from build123d import *

# Parameters (mm, degrees)
BOSS_EXTRUDE1_DEPTH = 6.35
SKETCH2_R           = 1.27
CUT_EXTRUDE1_DEPTH  = 397.811495062
SKETCH5_R           = 1.27
CUT_EXTRUDE2_DEPTH  = 397.811495062
SKETCH6_W           = 38.1
SKETCH6_H           = 7.62
CUT_EXTRUDE5_DEPTH  = 397.811495062
CUT_EXTRUDE9_DEPTH  = 397.811495062
SKETCH15_W          = 22.606
SKETCH15_H          = 12.446
CUT_EXTRUDE12_DEPTH = 397.811495062
SKETCH17_R          = 1.1
CUT_EXTRUDE13_DEPTH = 343.418665957
SKETCH18_R          = 1.5875
SKETCH18_R_2        = 1.5
SKETCH18_R_3        = 1.651
CUT_EXTRUDE14_DEPTH = 343.36317383
SKETCH19_R          = 1.65
CUT_EXTRUDE15_DEPTH = 343.36317383
SKETCH20_R          = 11.43
CUT_EXTRUDE16_DEPTH = 397.811495062
SKETCH24_R          = 1.905
CUT_EXTRUDE20_DEPTH = 343.36317383


with BuildPart() as part:
    # Sketch1 → Boss-Extrude1 (new body)
    with BuildSketch(Plane(origin=(0, 0, 0), x_dir=(1, 0, 0), z_dir=(0, 1, 0))):
        with BuildLine():
            Line((-203.2, 0), (-50.8, 0))
            ThreePointArc((-50.8, 0), (-14.878975516, 14.878975516), (0, 50.8))
            Line((0, 50.8), (0, 132.097510542))
            add(Edge.make_bspline(
                [(0, 132.097510542), (-11.235039637, 303.015237559), (-127, 304.8)],
                knots=[0.173908828, 0.173908828, 0.173908828, 0.982925822, 0.982925822, 0.982925822], degree=2))
            add(Edge.make_bspline(
                [(-254, 132.097510542), (-242.764960363, 303.015237559), (-127, 304.8)],
                knots=[0.173908828, 0.173908828, 0.173908828, 0.982925822, 0.982925822, 0.982925822], degree=2))
            Line((-254, 132.097510542), (-254, 50.8))
            ThreePointArc((-254, 50.8), (-239.121024484, 14.878975516), (-203.2, 0))
        make_face()
    extrude(amount=BOSS_EXTRUDE1_DEPTH)

    # Sketch2 → Cut-Extrude1 (cut, through all)
    with BuildSketch(Plane(origin=(0, 6.35, 0), x_dir=(1, 0, 0), z_dir=(0, 1, 0))):
        with Locations(Location((-135.34380131, 269.24, 0), (0, 0, 270))):
            Circle(SKETCH2_R)
    extrude(amount=-CUT_EXTRUDE1_DEPTH, mode=Mode.SUBTRACT)

    # Sketch5 → Cut-Extrude2 (cut, through all)
    with BuildSketch(Plane(origin=(0, 6.35, 0), x_dir=(1, 0, 0), z_dir=(0, 1, 0))):
        with Locations(Location((-119.59580131, 269.24, 0), (0, 0, 270))):
            Circle(SKETCH5_R)
    extrude(amount=-CUT_EXTRUDE2_DEPTH, mode=Mode.SUBTRACT)

    # Sketch6 → Cut-Extrude5 (cut, through all)
    with BuildSketch(Plane(origin=(0, 6.35, 0), x_dir=(1, 0, 0), z_dir=(0, 1, 0))):
        with Locations((-158.75, 207.01)):
            Rectangle(SKETCH6_W, SKETCH6_H)
        with Locations((-158.75, 260.35)):
            Rectangle(SKETCH6_W, SKETCH6_H)
        with Locations((-95.25000011, 207.01)):
            Rectangle(SKETCH6_W, SKETCH6_H)
        with Locations((-95.25000011, 260.35)):
            Rectangle(SKETCH6_W, SKETCH6_H)
    extrude(amount=-CUT_EXTRUDE5_DEPTH, mode=Mode.SUBTRACT)

    # Sketch12 → Cut-Extrude9 (cut, through all)
    with BuildSketch(Plane(origin=(0, 6.35, 0), x_dir=(1, 0, 0), z_dir=(0, 1, 0))):
        with BuildLine():
            Line((-152.4, 125.095), (-101.6, 125.095))
            ThreePointArc((-101.6, 125.095), (-99.695, 127), (-101.6, 128.905))
            Line((-101.6, 128.905), (-152.4, 128.905))
            ThreePointArc((-152.4, 128.905), (-154.305, 127), (-152.4, 125.095))
        make_face()
        Polygon((-159.512, 101.6), (-159.512, 88.9), (-145.203610871, 88.9), (-94.5, 88.9), (-94.5, 101.6), align=None)
    extrude(amount=-CUT_EXTRUDE9_DEPTH, mode=Mode.SUBTRACT)

    # Sketch15 → Cut-Extrude12 (cut, through all)
    with BuildSketch(Plane(origin=(0, 6.35, 0), x_dir=(1, 0, 0), z_dir=(0, 1, 0))):
        with Locations((-127.000000055, 25.4)):
            Rectangle(SKETCH15_W, SKETCH15_H)
    extrude(amount=-CUT_EXTRUDE12_DEPTH, mode=Mode.SUBTRACT)

    # Sketch17 → Cut-Extrude13 (cut, through all)
    with BuildSketch(Plane(origin=(-70.897607534, -2.5, -15.584277619), x_dir=(1, 0, 0), z_dir=(0, -1, 0))):
        with Locations(Location((-70.055392521, -9.692722381, 0), (0, 0, 270))):
            Circle(SKETCH17_R)
        with Locations(Location((-42.255392521, -9.692722381, 0), (0, 0, 90))):
            Circle(SKETCH17_R)
    extrude(amount=-CUT_EXTRUDE13_DEPTH, mode=Mode.SUBTRACT)

    # Sketch18 → Cut-Extrude14 (cut, through all)
    with BuildSketch(Plane(origin=(-70.897607534, 6.35, -15.584277619), x_dir=(1, 0, 0), z_dir=(0, -1, 0))):
        with Locations(Location((-108.366177987, -107.537321923, 0), (0, 0, 270))):
            Circle(SKETCH18_R)
        with Locations(Location((-156.626177987, -108.807321923, 0), (0, 0, 270))):
            Circle(SKETCH18_R)
        with Locations(Location((-141.386177987, -159.607321923, 0), (0, 0, 270))):
            Circle(SKETCH18_R)
        with Locations(Location((-113.446177987, -159.607321923, 0), (0, 0, 270))):
            Circle(SKETCH18_R)
        with Locations(Location((-36.13742283, -36.50630685, 0), (0, 0, 270))):
            Circle(SKETCH18_R_2)
        with Locations(Location((-76.13742283, -55.50630685, 0), (0, 0, 270))):
            Circle(SKETCH18_R_2)
        with Locations(Location((-82.468497304, -27.730722381, 0), (0, 0, 270))):
            Circle(SKETCH18_R_3)
        with Locations(Location((-29.128497304, -27.730722381, 0), (0, 0, 270))):
            Circle(SKETCH18_R_3)
    extrude(amount=CUT_EXTRUDE14_DEPTH, mode=Mode.SUBTRACT)

    # Sketch19 → Cut-Extrude15 (cut, through all)
    with BuildSketch(Plane(origin=(-70.897607534, 0, -15.584277619), x_dir=(1, 0, 0), z_dir=(0, -1, 0))):
        with Locations(Location((-176.212392466, -65.014477652, 0), (0, 0, 270))):
            Circle(SKETCH19_R)
        with Locations(Location((-157.162392466, -65.014477652, 0), (0, 0, 270))):
            Circle(SKETCH19_R)
        with Locations(Location((-176.212392466, -86.714477652, 0), (0, 0, 270))):
            Circle(SKETCH19_R)
        with Locations(Location((-157.162392466, -86.714477652, 0), (0, 0, 270))):
            Circle(SKETCH19_R)
        with Locations(Location((64.007607534, -86.714477652, 0), (0, 0, 270))):
            Circle(SKETCH19_R)
        with Locations(Location((44.957607534, -86.714477652, 0), (0, 0, 270))):
            Circle(SKETCH19_R)
        with Locations(Location((44.957607534, -65.014477652, 0), (0, 0, 270))):
            Circle(SKETCH19_R)
        with Locations(Location((64.007607534, -65.014477652, 0), (0, 0, 270))):
            Circle(SKETCH19_R)
    extrude(amount=-CUT_EXTRUDE15_DEPTH, mode=Mode.SUBTRACT)

    # Sketch20 → Cut-Extrude16 (cut, through all)
    with BuildSketch(Plane(origin=(0, 6.35, 0), x_dir=(1, 0, 0), z_dir=(0, 1, 0))):
        with Locations(Location((-53.826154214, 47.757613525, 0), (0, 0, 270))):
            Circle(SKETCH20_R)
        with Locations(Location((-203.77940498, 47.757613525, 0), (0, 0, 270))):
            Circle(SKETCH20_R)
    extrude(amount=-CUT_EXTRUDE16_DEPTH, mode=Mode.SUBTRACT)

    # Sketch24 → Cut-Extrude20 (cut, through all)
    with BuildSketch(Plane(origin=(-70.897607534, 0, -15.584277619), x_dir=(1, 0, 0), z_dir=(0, -1, 0))):
        with Locations(Location((-62.829392521, -23.916722381, 0), (0, 0, 270))):
            Circle(SKETCH24_R)
        with Locations(Location((-47.081392521, -23.916722381, 0), (0, 0, 270))):
            Circle(SKETCH24_R)
        with Locations(Location((-47.081392521, 4.531277619, 0), (0, 0, 270))):
            Circle(SKETCH24_R)
        with Locations(Location((-62.829392521, 4.531277619, 0), (0, 0, 270))):
            Circle(SKETCH24_R)
    extrude(amount=-CUT_EXTRUDE20_DEPTH, mode=Mode.SUBTRACT)


solid = part.part
Geometry: final body of the model. Coordinates: model frame, mm. A direction names the side the tool comes from. Round coordinates to 2 decimals unless told otherwise and drop trailing zeros. Write each question's results on one line, items separated by ' | '. Start each with the question number.
1) First-contact query: P1, Ø1.9, axis at x = -155.5, y = 4, coming from the -Z side; P2, Ø3, axis at y = 4.5, z = -236, coming from the +X side; P3, Ø3, axis at y = 3.5, z = -208.5, coming from the -X side. Flat tips, straight axial feed; report the tip coordinate or a pass-through.
2) Cut plane A-A on y = 1.75. Count the separate pieces of the cut face and the enclosed holes in it, then the cut area to 3 significant figures.
3) Mould query, pull axis Z, two halves, no side actions, for faces 3 (the face through (-159, 3, -210.82)), 4 (the face through (-239.514, 3.131, -15.276)), 5 (the face through (0, 3, -91)). Classes: released by +Z, released by -Z, zero draft, split by the parting line, or undercut.
4) Line query: probe 1 along Z at (x, y) = (-112, 4.5) (3 decimals); probe 2 along Z at (x, y) = (-166, 4.5); probe 3 along X at (y, z) = (2.75, -41). Output: solid intervals per line, ascending. Write a range as [from, to].
5) Access query for faces 1 (the face through (-127, 3, -101.6)), 2 (the face through (-128, 3, 0)). Directions: +Z, -Z, +X, -X, +Y, -Y. A direction counts if a zero-diameter tool reaches every point of the face in a straight line with its end or side. Return the directions, or none.
Verdict:
1) P1: stops at z = -301.66 | P2: stops at x = -22.2 | P3: stops at x = -241.85
2) separate pieces: 1 | enclosed holes: 33 | area: 64,100 mm2
3) face 3: undercut | face 4: released by +Z | face 5: zero draft
4) probe 1: z = [-303.807, -264.16], [-256.54, -210.82], [-203.2, -128.905], [-125.095, -101.6], [-88.9, 0] | probe 2: z = [-298.44, -264.16], [-256.54, -210.82], [-203.2, 0] | probe 3: x = [-253.05, -213], [-194.56, -134.9], [-132.55, -119.15], [-116.8, -63.04], [-44.61, -0.95]
5) face 1: +Y, -Y | face 2: +Z, +X, -X, +Y, -Y
